```python
from build123d import *

# Parameters (mm, degrees)
EXTRUDE_1_DEPTH     = 70
SKETCH_2_W          = 50
SKETCH_2_H          = 46.62381926
CUT_EXTRUDE_1_DEPTH = 70
CUT_EXTRUDE_2_REACH = 72
SKETCH_3_R          = 17.5
CUT_EXTRUDE_3_DEPTH = 70


with BuildPart() as part:
    # 草图1 → 凸台-拉伸1 (new body)
    with BuildSketch(Plane.XY):
        Polygon((-65.25, 63.25), (-65.25, -6.75), (-105.25, -50), (-105.25, -70), (194.75, -70), (194.75, 0), (124.75, 0), (124.75, -50), (24.75, -50), (-35.25, -6.75), (-35.25, 63.25), align=None)
    extrude(amount=EXTRUDE_1_DEPTH)

    # 草图2 → 切除-拉伸1 (cut)
    with BuildSketch(Plane.XY.offset(70)):
        with Locations((159.75, -36.68809037)):
            Rectangle(SKETCH_2_W, SKETCH_2_H)
    extrude(amount=-CUT_EXTRUDE_1_DEPTH, mode=Mode.SUBTRACT)

    # 草图3 → 切除-拉伸2 (cut, up to next)
    with BuildSketch(Plane(origin=(-35.25, 0, 0), x_dir=(0, 0, -1), z_dir=(1, 0, 0)), mode=Mode.PRIVATE) as cut_extrude_2_sk1:
        with Locations((-35, 43.25)):
            Circle(SKETCH_3_R)
    cut_extrude_2_tool1 = extrude(cut_extrude_2_sk1.sketch, amount=-CUT_EXTRUDE_2_REACH, mode=Mode.PRIVATE) & part.part
    add(cut_extrude_2_tool1.solids().sort_by_distance((-35.25, 43.25, 35))[0], mode=Mode.SUBTRACT)

    # 草图4 → 切除-拉伸3 (cut)
    with BuildSketch(Plane.XY.offset(70)):
        Polygon((-65.25, -25), (-90.25, -50), (-65.25, -50), align=None)
        Polygon((-35.25, -25), (-35.25, -50), (-5.25, -50), align=None)
    extrude(amount=-CUT_EXTRUDE_3_DEPTH, mode=Mode.SUBTRACT)


solid = part.part
```
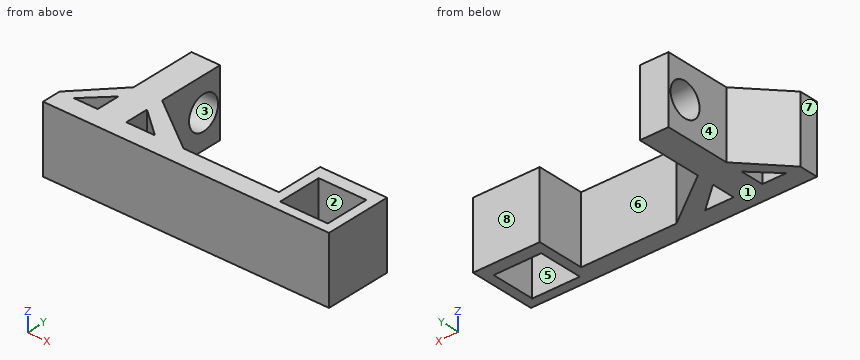
Check sheet for the modelled part. Datum: model origin and axes. Units: mm. Face numbers are marked on the shaded views. A direction names the side the tool comes from. Coordinates: 2 decimals unless noted, no trailing zeros. Order: outer loops, then holes, each group sorted by start corner. A loop starts at its lowest first (then second) coordinate and runs counter-clockwise, first axis right, second up. Notation, with made-up numbers: M 2.25,60.25 L 33.25,60.25 A14 ccw 33.25,67.25 Z; hole C 70.5,76.5 d10. An arc over 180 degrees is marked long. Write each question's results on one line, items separated by ' | '. Start each with the question number.
1. Access from +Z, -Z, +X, -X, +Y, -Y to the whole of each face (thin tool, end or side, straight path). Record for the marked faces 4, 5, 6, 7 and 8.
2. Cross-section at C-C on x = -81.5. Record the cut outline in (y, z), and give its area (3 significant figures).
3. Cross-section at D-D on z = 63.5. Record the cut outline in (x, y).
4. Cross-section at A-A on z = 35. Record the cut outline in (x, y), and give its area (3 significant figures).
5. Cross-section at B-B on y = 43.25. Record the cut outline in (x, z).
6. Go/stop test with flat-tipped pins: P1, Ø21, axis at y = 39, z = 25, coming from the +X side; P2, Ø2, axis at y = 29, z = 53.5, coming from the -X side; P3, Ø9, axis at x = -14, z = 23.5, coming from the +Y side. Record where each tip stops, or that it passes through.
7. Material ranges on probe 1 along Y at (x, z) = (144.5, 5.5); probe 2 along Z at (x, y) = (-43, 43); probe 3 along X at (y, z) = (-19.5, 45), recorded low to high.
8. Mould release check, pull along Z, two halves, no side actions. Record for the marked faces 1, 2 and 3: +Z half, -Z half, draft (parallel to the pull), parting line (faces both ways), or undercut.
Checks:
1) face 4: +Z, -Z, -X, +Y | face 5: +Z, -Z | face 6: +Z, -Z, +Y | face 7: +Z, -Z, -X, +Y, -Y | face 8: +Z, -Z, +X, +Y
2) outline: M -70,0 L -50,0 L -50,70 L -70,70 Z; M -41.25,0 L -24.32,0 L -24.32,70 L -41.25,70 Z | area: 2,590 mm²
3) outline: M -105.25,-70 L 194.75,-70 L 194.75,0 L 124.75,0 L 124.75,-50 L 24.75,-50 L -35.25,-6.75 L -35.25,63.25 L -65.25,63.25 L -65.25,-6.75 L -105.25,-50 Z; hole M -90.25,-50 L -65.25,-50 L -65.25,-25 Z; hole M -35.25,-50 L -5.25,-50 L -35.25,-25 Z; hole M 134.75,-60 L 184.75,-60 L 184.75,-13.38 L 134.75,-13.38 Z
4) outline: M -105.25,-70 L 194.75,-70 L 194.75,0 L 124.75,0 L 124.75,-50 L 24.75,-50 L -35.25,-6.75 L -35.25,25.75 L -65.25,25.75 L -65.25,-6.75 L -105.25,-50 Z; M -65.25,60.75 L -35.25,60.75 L -35.25,63.25 L -65.25,63.25 Z; hole M -90.25,-50 L -65.25,-50 L -65.25,-25 Z; hole M -35.25,-50 L -5.25,-50 L -35.25,-25 Z; hole M 134.75,-60 L 184.75,-60 L 184.75,-13.38 L 134.75,-13.38 Z | area: 11,000 mm²
5) outline: M -65.25,0 L -35.25,0 L -35.25,17.5 L -65.25,17.5 Z; M -65.25,52.5 L -35.25,52.5 L -35.25,70 L -65.25,70 Z
6) P1: stops at x = -35.25 | P2: stops at x = -65.25 | P3: stops at y = -18.82
7) probe 1: y = -70 to -60, -13.38 to 0 | probe 2: z = 0 to 17.5, 52.5 to 70 | probe 3: x = -77.04 to -17.56, 124.75 to 134.75, 184.75 to 194.75
8) face 1: -Z half | face 2: draft | face 3: undercut
